from build123d import *

# Parameters (mm, degrees)
MODEL_R             = 1.3
MODEL_R_2           = 1.5
BOSS_EXTRUDE1_DEPTH = 3


with BuildPart() as part:
    # Model → Boss-Extrude1 (new body)
    with BuildSketch(Plane.XY):
        with BuildLine():
            ThreePointArc((14.161227702, 11.70429003), (14.127993258, 6.180717338), (19.644033131, 5.890434821))
            ThreePointArc((19.644033131, 5.890434821), (27.067718512, 9.016008339), (34.921377151, 7.227053216))
            ThreePointArc((34.921377151, 7.227053216), (35.664878745, 6.883684708), (36.462728707, 6.698936254))
            ThreePointArc((36.462728707, 6.698936254), (39.928001734, 7.988038053), (40.861936188, 11.565420761))
            ThreePointArc((40.861936188, 11.565420761), (37.563797473, 30.440091822), (40.733692306, 49.336723623))
            ThreePointArc((40.733692306, 49.336723623), (37.814731301, 54.297590711), (32.991594421, 51.15627152))
            ThreePointArc((32.991594421, 51.15627152), (26.788825125, 29.897000757), (14.161227702, 11.70429003))
        make_face()
        with Locations((36.961607348, 50.667664276)):
            Circle(MODEL_R, mode=Mode.SUBTRACT)
        with Locations((17.037547355, 8.924717563)):
            Circle(MODEL_R_2, mode=Mode.SUBTRACT)
        with Locations((36.961484604, 10.667620763)):
            Circle(MODEL_R_2, mode=Mode.SUBTRACT)
    extrude(amount=BOSS_EXTRUDE1_DEPTH)


solid = part.part
Check sheet for the modelled part. Datum: model origin and axes. Units: mm. A direction names the side the tool comes from. Round coordinates to 2 decimals unless told otherwise and drop trailing zeros. Loops run counter-clockwise (first coordinate to the right, second up) from the corner with the lowest first, then second, coordinate; pieces in that order, holes last. Notation, with made-up numbers: (-26.5, -13.75) -> (-11.5, -13.75) arc R16 cw to (-11.5, 6.25) -> close; hole circle Ø9 at (10, 59.5). An arc over 180 degrees is marked (long way). Put each result on its own line as item: value. Start each with the question number.
1. Access from +Z, -Z, +X, -X, +Y, -Y to the whole of each face (thin tool, end or side, straight path). Record for faces 1 (the face through (35.65, 6.89, 1.48)), 2 (the face through (30, 25, 0)).
2. Gauge pin test, flat ends, axial feed: pin 1 (1 mm diameter, centred on y = 19, z = 1.5, fed in from +X); pin 2 (2.5 mm diameter, centred on x = 36.96, y = 50.67, fed in from -Z); pin 3 (1.5 mm diameter, centred on y = 18, z = 1, fed in from +X); pin 4 (1.5 mm diameter, centred on y = 31, z = 1, fed in from +X). Record the tip position at first contact, or that the pin passes through.
3. Section check C-C (y = 19). Enter the section's corners in (x, z).
4. Section check D-D (x = 25). Enter the section's corners in (y, z), plus the area to 3 significant figures.
5. Scan lines: probe 1 along Y at (x, z) = (36, 1.1); probe 2 along Y at (x, z) = (16.75, 1.8); probe 3 along X at (y, z) = (7, 2.2). Record each from-to range of solid material in increasing order.
6. Section check A-A (x = 16.5). Enter the section's corners in (y, z).
7. Section check B-B (z = 1.5). Enter the section's corners in (x, y).
Findings:
1. face 1: +Z, -Z, -Y
1. face 2: -Z, +X, -X, +Y, -Y
2. pin 1: stops at x = 38.88
2. pin 2: passes through
2. pin 3: stops at x = 39.16
2. pin 4: stops at x = 37.57
3. outline: (20.29, 0) -> (38.77, 0) -> (38.77, 3) -> (20.29, 3) -> close
4. outline: (8.67, 0) -> (26.41, 0) -> (26.41, 3) -> (8.67, 3) -> close
4. area: 53.2 mm^2
5. probe 1: y = 6.78 to 9.52, 11.82 to 49.79, 51.54 to 54.3
5. probe 2: y = 4.94 to 7.45, 10.4 to 14.54
5. probe 3: x = 13.53 to 21.14, 35.37 to 38.55
6. outline: (4.96, 0) -> (7.52, 0) -> (7.52, 3) -> (4.96, 3) -> close; (10.33, 0) -> (14.25, 0) -> (14.25, 3) -> (10.33, 3) -> close
7. outline: (14.16, 11.7) arc R4 ccw to (19.64, 5.89) arc R13.15 cw to (34.92, 7.23) arc R4 ccw to (36.46, 6.7) arc R4.01 ccw to (40.86, 11.57) arc R56.76 cw to (40.73, 49.34) arc R3.98 ccw (long way) to (32.99, 51.16) arc R68.89 cw to start; hole circle Ø3 at (17.04, 8.92); hole circle Ø3 at (36.96, 10.67); hole circle Ø2.6 at (36.96, 50.67)
